CAD build for the part. Positions are in the model's coordinates, mm. A direction names the side the tool comes from. Coordinates: 2 decimals unless noted, no trailing zeros. Write item = value, one per line. Start each with the question number.
(1) Pull direction Y, two halves, no side cores. Call faces 3 (the face through (-0.925, -25.733, 3.507)), 4 (the face through (14, 35, 3)), 5 (the face through (0, -2, 3)), 6 (the face through (-0.2, 47.28, 1.73)): +Y half, -Y half, draft (parallel to the pull), parting line (faces both ways), or undercut.
(2) Flat gauge pins, fed straight in: P1, Ø1.5, axis at x = -11, z = 1.5, coming from the +Y side; P2, Ø1, axis at y = -38.5, z = 0.5, coming from the -X side; P3, Ø1.5, axis at y = 27.5, z = 3, coming from the +X side. Where does each tip first touch, or does it go through?
(3) Tool access for faces 1 (the face through (-1, 1, 0)), 2 (the face through (-0.196, 16.892, 2.493)): list every direction of +Z, -Z, +X, -X, +Y, -Y with a clear straight run to the whole face (end or side of a thin tool).
(4) Drill centre lines: line 1 (X direction, y = 32, z = 2.4); line 2 (Z direction, x = -2, y = 45.5); line 3 (Y direction, x = 30.5, z = 2.85). Where is each one in solid material? Low to high. Write a range as from..to.
```python
from build123d import *

# Parameters (mm, degrees)
F0_R     = 50
F1_DEPTH = 4
F2_R     = 25.75
F3_DEPTH = 1
F5_DEPTH = 2
F6_SIZE2 = 3.732041
F6_SIZE  = 0.99999


# Not quite as in the source:
# - a fillet or chamfer is up to 0.001 mm smaller than in the source, because OpenCascade refuses the exact size
# - a feature names something its author has since deleted; it is built from what else it names


with BuildPart() as f1:
    # F0 (on Top) → F1 (new body)
    with BuildSketch(Plane.XY):
        Circle(F0_R)
    extrude(amount=F1_DEPTH)

    # F2 (on face) → F3 (cut)
    with BuildSketch(Plane.XY.offset(4)):
        Circle(F2_R)
    extrude(amount=-F3_DEPTH, mode=Mode.SUBTRACT)

    # F4 (on face) → F5 (cut)
    with BuildSketch(Plane.XY.offset(4)):
        with BuildLine():
            Line((-14, 21.6116288141), (-14, 15))
            Line((-14, 15), (14, 15))
            Line((14, 15), (14, 21.6116288141))
            ThreePointArc((14, 21.6116288141), (0, 25.75), (-14, 21.6116288141))
        make_face()
        with BuildLine():
            Line((-14, 48), (-14, 21.6116288141))
            ThreePointArc((-14, 21.6116288141), (0, 25.75), (14, 21.6116288141))
            Line((14, 21.6116288141), (14, 48))
            ThreePointArc((14, 48), (0, 50), (-14, 48))
        make_face()
        with BuildLine():
            Line((-14, 55), (-14, 48))
            ThreePointArc((-14, 48), (0, 50), (14, 48))
            Line((14, 48), (14, 55))
            Line((14, 55), (-14, 55))
        make_face()
    extrude(amount=-F5_DEPTH, mode=Mode.SUBTRACT)

    # F6 (size 1 and 3.7320508076 in the source; OpenCascade refuses exactly that, so slightly less here)
    f6_edges = [f1.edges().sort_by_distance(p)[0] for p in [
        (0, 15, 2),
        (-30, -40, 4),
        (0, 50, 2),
        (40, 30, 4),
    ]]
    chamfer(f6_edges, length=F6_SIZE, length2=F6_SIZE2)


solid = f1.part
```
Findings below:
q1.face_3 = undercut
q1.face_4 = draft
q1.face_5 = undercut
q1.face_6 = +Y half
q2.P1 = 48.9
q2.P2 = -32.5
q2.P3 = 42.24
q3.face_1 = -Z, +X, -X, +Y, -Y
q3.face_2 = +Z, +Y
q4.line_1 = -38.42..-14, 14..38.42
q4.line_2 = 0..2
q4.line_3 = -39.62..39.62
